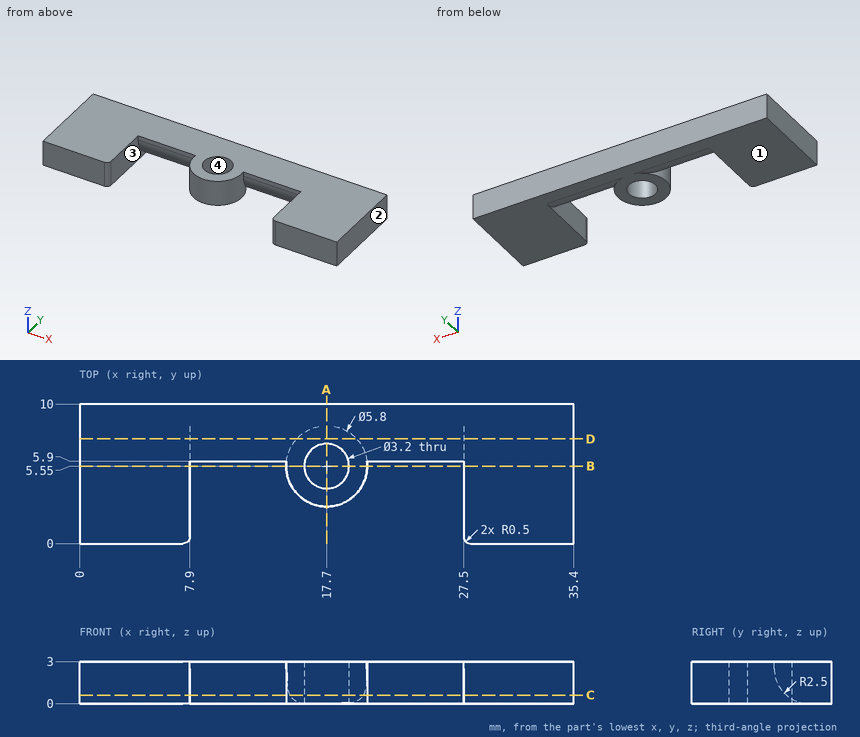
Print and shaded views of the part. All mm, measured from the part's lowest x, y and z. Give positions to 0.01 mm unless a question says otherwise; leave off trailing zeros. Loops run counter-clockwise (first coordinate to the right, second up) from the corner with the lowest first, then second, coordinate; pieces in that order, holes last. Notation, with made-up numbers: (-15.75, 66) -> (38.25, 66) arc R14 ccw to (38.25, 82) -> close; hole circle Ø6 at (32.25, 82). An arc over 180 degrees is marked (long way). One line per question, with ' | ' between items. Start each with the question number.
1) Cut at C-C (z = 0.6). Give the cut face in (x, y).
2) Cut at B-B (y = 5.55). Give the cut face in (x, z).
3) Pin check, flat tip, straight feed: pin 1 (1.5 mm diameter, centred on x = 23, z = 1.5, fed in from -Y). Stop position of the tip, or through.
4) Two-plate mould, pull along X, no slides. Class the marked faces 1, 2, 3 and 4: released by +X, released by -X, zero draft, split by the parting line, or undercut.
5) Probe L1, parallel to X at y = 1, z = 1.6; L2, parallel to Y at x = 17.7, z = 1.75; L3, parallel to X at y = 3, z = 0.6. List the from-to ranges inside material, lowest first.
6) Cut at A-A (x = 17.7). Give the cut face in (y, z), plus the area to 4 significant figures.
7) Cut at D-D (y = 7.5). Give the cut face in (x, z).
Return value:
1) outline: (0, 0) -> (7.4, 0) arc R0.5 ccw to (7.9, 0.5) -> (7.9, 6.78) -> (15.07, 6.78) arc R2.9 ccw (long way) to (20.33, 6.78) -> (27.5, 6.78) -> (27.5, 0.5) arc R0.5 ccw to (28, 0) -> (35.4, 0) -> (35.4, 10) -> (0, 10) -> close; hole circle Ø3.2 at (17.7, 5.55)
2) outline: (0, 0) -> (7.9, 0) -> (7.9, 3) -> (0, 3) -> close; (14.8, 0) -> (16.1, 0) -> (16.1, 3) -> (14.8, 3) -> close; (19.3, 0) -> (20.6, 0) -> (20.6, 3) -> (19.3, 3) -> close; (27.5, 0) -> (35.4, 0) -> (35.4, 3) -> (27.5, 3) -> close
3) pin 1: y = 5.91
4) face 1: zero draft | face 2: released by +X | face 3: undercut | face 4: undercut
5) L1: 0 to 7.9, 27.5 to 35.4 | L2: 2.65 to 3.95, 7.15 to 10 | L3: 0 to 7.9, 16.32 to 19.08, 27.5 to 35.4
6) outline: (2.65, 0) -> (3.95, 0) -> (3.95, 3) -> (2.65, 3) -> close; (7.15, 0) -> (10, 0) -> (10, 3) -> (7.15, 3) -> close | area: 12.45 mm^2
7) outline: (0, 0) -> (7.9, 0) -> (7.9, 0.17) -> (15.55, 0.17) -> (15.55, 0) -> (19.85, 0) -> (19.85, 0.17) -> (27.5, 0.17) -> (27.5, 0) -> (35.4, 0) -> (35.4, 3) -> (0, 3) -> close
